Can you work these out from the model? Positions are in its coordinate system, mm. A direction names the side the tool comes from. Give positions to 0.01 mm unless a question says otherwise; leave off trailing zeros. Order: outer loops, then holes, each group sorted by start corner. A loop starts at its lowest first (then second) coordinate and runs counter-clockwise, first axis right, second up. Notation, with made-up numbers: M 64,35.25 L 69,35.25 A7 cw 69,48.25 Z; hole C 11,70.5 d6. An arc over 180 degrees is marked long. Answer as a JSON object with one key per item and string values.
```python
from build123d import *

# Parameters (mm, degrees)
SKETCH1_R           = 1.5875
BOSS_EXTRUDE1_DEPTH = 1.27
CUT_EXTRUDE1_DEPTH  = 2.54


with BuildPart() as part:
    # Sketch1 → Boss-Extrude1 (new body)
    # profile 1 of 5: a face of its own
    with BuildSketch(Plane(origin=(0, 0, 0), x_dir=(1, 0, 0), z_dir=(0, 1, 0))):
        with BuildLine():
            ThreePointArc((-3.549757914, -3.175), (-4.7625, 0), (-3.549757914, 3.175))
            Line((-3.549757914, 3.175), (-19.05, 3.175))
            Line((-19.05, 3.175), (-19.05, -3.175))
            Line((-19.05, -3.175), (-3.549757914, -3.175))
        make_face()
        with Locations(Location((-15.875, 0, 0), (0, 0, 270))):
            Circle(SKETCH1_R, mode=Mode.SUBTRACT)
    # profile 2 of 5: a face of its own
    with BuildSketch(Plane(origin=(0, 0, 0), x_dir=(1, 0, 0), z_dir=(0, 1, 0))):
        with BuildLine():
            Line((0, -3.175), (0, 0))
            Line((0, 0), (0, 3.175))
            Line((0, 3.175), (-3.549757914, 3.175))
            ThreePointArc((-3.549757914, 3.175), (-4.7625, 0), (-3.549757914, -3.175))
            Line((-3.549757914, -3.175), (0, -3.175))
        make_face()
    # profile 3 of 5: a face of its own
    with BuildSketch(Plane(origin=(0, 0, 0), x_dir=(1, 0, 0), z_dir=(0, 1, 0))):
        with BuildLine():
            Line((0, 3.175), (0, 0))
            Line((0, 0), (0, -3.175))
            Line((0, -3.175), (-3.549757914, -3.175))
            ThreePointArc((-3.549757914, -3.175), (1.699365203, -4.44899586), (4.7625, 0))
            ThreePointArc((4.7625, 0), (1.699365203, 4.44899586), (-3.549757914, 3.175))
            Line((-3.549757914, 3.175), (0, 3.175))
        make_face()
    # profile 4 of 5: a face of its own
    with BuildSketch(Plane(origin=(0, 0, 0), x_dir=(1, 0, 0), z_dir=(0, 1, 0))):
        with BuildLine():
            Line((0, -3.175), (0, 0))
            Line((0, 0), (0, 3.175))
            Line((0, 3.175), (-3.549757914, 3.175))
            ThreePointArc((-3.549757914, 3.175), (-4.7625, 0), (-3.549757914, -3.175))
            Line((-3.549757914, -3.175), (0, -3.175))
        make_face()
    # profile 5 of 5: a face of its own
    with BuildSketch(Plane(origin=(0, 0, 0), x_dir=(1, 0, 0), z_dir=(0, 1, 0))):
        with BuildLine():
            Line((0, 3.175), (0, 0))
            Line((0, 0), (0, -3.175))
            Line((0, -3.175), (-3.549757914, -3.175))
            ThreePointArc((-3.549757914, -3.175), (1.699365203, -4.44899586), (4.7625, 0))
            ThreePointArc((4.7625, 0), (1.699365203, 4.44899586), (-3.549757914, 3.175))
            Line((-3.549757914, 3.175), (0, 3.175))
        make_face()
    extrude(amount=BOSS_EXTRUDE1_DEPTH)

    # Sketch2 → Cut-Extrude1 (cut)
    with BuildSketch(Plane(origin=(0, 1.27, 0), x_dir=(1, 0, 0), z_dir=(0, 1, 0))):
        Polygon((3.666174209, 0), (1.833087105, 3.175), (-1.833087105, 3.175), (-3.666174209, 0), (-1.833087105, -3.175), (1.833087105, -3.175), align=None)
    extrude(amount=-CUT_EXTRUDE1_DEPTH, mode=Mode.SUBTRACT)


solid = part.part
```
1) I want a section at A-A on z = -1.25. Write out the boundary of the cut face in (x, y).
Results found:
{"outline": "M -19.05,0 L -16.85,0 L -16.85,1.27 L -19.05,1.27 Z; M -14.9,0 L -2.94,0 L -2.94,1.27 L -14.9,1.27 Z; M 2.94,0 L 4.6,0 L 4.6,1.27 L 2.94,1.27 Z"}
2) I want a section at B-B on y = 0.7. Count the separate pieces of the cut face and the enclosed holes in it, and give its area (3 significant figures).
Results found:
{"separate pieces": "1", "enclosed holes": "2", "area": "122 mm²"}
3) Thinking about a two-plate mould opening in Z: for faces 4 (the face through (0, 1, 3.175)), 5 (the face through (-7, 1.27, 0)), 6 (the face through (-17.425, 0.626, -0.344)), 7 (the face through (-11, 1, -3.175)), which applies, pulls with the +Z half, pulls with the -Z half, needs draft (parallel to the pull), parting line crosses it, or undercut?
Results found:
{"face 4": "undercut", "face 5": "needs draft", "face 6": "undercut", "face 7": "pulls with the -Z half"}
4) For faces 1 (the face through (2.737, 0.644, 1.61)), 2 (the face through (-11, 1, 3.175)), 3 (the face through (-7, 0, 0)), which set-ups out of +Z, -Z, +X, -X, +Y, -Y let a thin tool reach every point of the face, with its end or its side?
Results found:
{"face 1": "+Y, -Y", "face 2": "+Z, -X, +Y, -Y", "face 3": "+Z, -Z, +X, -X, -Y"}
5) I want a section at C-C on x = -10. Write out the boundary of the cut face in (y, z) (3 decimals), and give its area (3 significant figures).
Results found:
{"outline": "M 0,-3.175 L 1.27,-3.175 L 1.27,3.175 L 0,3.175 Z", "area": "8.06 mm²"}
6) I need wall thicknesses on L1, parallel to Z at x = -7.75, y = 0.3 (3 decimals); L2, parallel to Z at x = 0.25, y = 0.2 (3 decimals); L3, parallel to Z at x = -17.25, y = 0.7 (3 decimals). Which ranges of each line are inside material? Lowest first, please.
Results found:
{"L1": "z = -3.175 to 3.175", "L2": "z = -4.756 to -3.175, 3.175 to 4.756", "L3": "z = -3.175 to -0.793, 0.793 to 3.175"}
7) I'm going to push a flat-ended pin straight in: pin 1 Ø2.5 at (x, z) = (-15.875, 0) entering from -Y. Where does the tip first touch, or does it pass through?
Results found:
{"pin 1": "passes through"}
